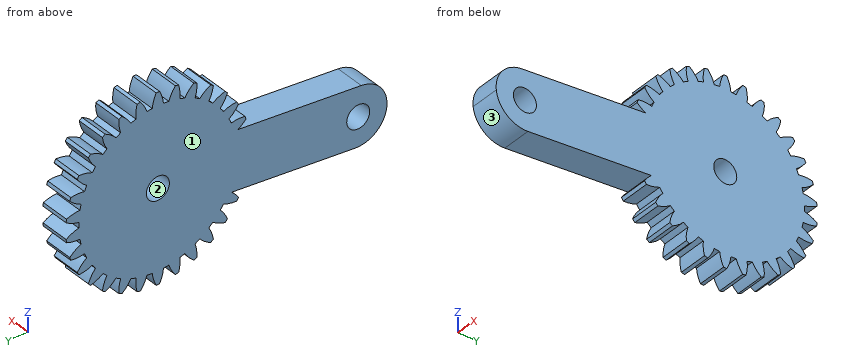
```python
from build123d import *

# Parameters (mm, degrees)
BASPROSKE_W         = 5
BASPROSKE_H         = 16
TOOTHCUT_DEPTH      = 24.173260453
TEETHCUTS_COUNT     = 30
TEETHCUTS_ANGLE     = 348
BORSKE_R            = 0.4
BORE_DEPTH          = 50.0000508
SKETCH1_R           = 2
BOSS_EXTRUDE1_DEPTH = 5
SKETCH2_R           = 2
CUT_EXTRUDE1_DEPTH  = 44.650585033
FILLET1_R           = 5


with BuildPart() as part:
    # BasProSke → Base-Revolve (revolve)
    with BuildSketch(Plane(origin=(0, 0, 0), x_dir=(1, 0, 0), z_dir=(0, 1, 0)), mode=Mode.PRIVATE) as base_revolve_sk:
        with Locations((2.5, 8)):
            Rectangle(BASPROSKE_W, BASPROSKE_H)
    revolve(base_revolve_sk.sketch.rotate(Axis((-10, 0, 0), (1, 0, 0)), 180), axis=Axis((-10, 0, 0), (1, 0, 0)))

    # TooCutSke → ToothCut (cut, through all)
    with BuildSketch(Plane(origin=(0, 0, 0), x_dir=(0, 0, -1), z_dir=(1, 0, 0))):
        with BuildLine():
            ThreePointArc((0.466400716, 13.741086979), (0, 13.749), (-0.466400716, 13.741086979))
            ThreePointArc((-0.466400716, 13.741086979), (-0.819142092, 14.899954875), (-1.3974676, 15.964351834))
            ThreePointArc((-1.3974676, 15.964351834), (0, 16.0254), (1.3974676, 15.964351834))
            ThreePointArc((1.3974676, 15.964351834), (0.819142092, 14.899954875), (0.466400716, 13.741086979))
        make_face()
    toothcut = extrude(amount=TOOTHCUT_DEPTH, mode=Mode.SUBTRACT)

    # TeethCuts: ToothCut ×30 about axis
    teethcuts_axis = Axis((-10, 0, 0), (1, 0, 0))
    for i in range(1, TEETHCUTS_COUNT):
        add(toothcut.rotate(teethcuts_axis, i * TEETHCUTS_ANGLE / (TEETHCUTS_COUNT - 1)), mode=Mode.SUBTRACT)

    # BorSke → Bore (cut, symmetric)
    with BuildSketch(Plane(origin=(0, 0, 0), x_dir=(0, 0, -1), z_dir=(1, 0, 0))):
        with Locations(Location((0, 0, 0), (0, 0, 180))):
            Circle(BORSKE_R)
    extrude(amount=BORE_DEPTH, both=True, mode=Mode.SUBTRACT)

    # Sketch1 → Boss-Extrude1 (add)
    with BuildSketch(Plane(origin=(5, 0, 0), x_dir=(0, 0, -1), z_dir=(1, 0, 0))):
        Polygon((4.972609477, 0.522642316), (9.153748008, -39.258233498), (-0.791470946, -40.303518131), (-4.972609477, -0.522642316), align=None)
        with Locations((3.658496214, -34.808266338)):
            Circle(SKETCH1_R, mode=Mode.SUBTRACT)
    extrude(amount=-BOSS_EXTRUDE1_DEPTH)

    # Sketch2 → Cut-Extrude1 (cut, through all)
    with BuildSketch(Plane(origin=(5, 0, 0), x_dir=(0, 0, -1), z_dir=(1, 0, 0))):
        Circle(SKETCH2_R)
    extrude(amount=-CUT_EXTRUDE1_DEPTH, mode=Mode.SUBTRACT)

    # Fillet1
    fillet1_edges = [part.edges().sort_by_distance(p)[0] for p in [
        (2.5, -39.258233498, -9.153748008),
        (2.5, -40.303518131, 0.791470946),
    ]]
    fillet(fillet1_edges, radius=FILLET1_R - 0.0001)  # a hair under: the kernel refuses the full size


solid = part.part
```
Here's how the part is built. I have some questions about the finished solid (model axes, mm). Face numbers are marked on the shaded views. Coordinates: 2 decimals unless noted, no trailing zeros. Order: outer loops, then holes, each group sorted by start corner. A loop starts at its lowest first (then second) coordinate and runs counter-clockwise, first axis right, second up. Notation, with made-up numbers: (80, 41.5) -> (133, 41.5) arc R16 ccw to (133, 66.5) -> close; hole circle Ø7 at (44, 25). An arc over 180 degrees is marked (long way). Return JSON: item names as keys, results as strings.
1) If we section it at A-A on x = 3.2: State how many separate pieces and enclosed holes the cut face has, plus the area to 3 significant figures.
Conclusion:
{"separate pieces": "1", "enclosed holes": "2", "area": "910 mm²"}
2) I'm going to push flat-ended pins straight in: P1, Ø3, axis at x = 1, y = 2.5, coming from the +Z side; P2, Ø2, axis at x = 2, z = 7, coming from the +Y side; P3, Ø3, axis at y = 0, z = 0, coming from the +X side. Where does each tip first touch, or does it pass through?
Conclusion:
{"P1": "stops at z = 15.71", "P2": "stops at y = 14", "P3": "passes through"}
3) If I drill on probe 1 along Y at (x, z) = (2.9, 14); probe 2 along Z at (x, y) = (0.3, -12); probe 3 along Y at (x, z) = (1.5, 0), over which ranges is the centre line in solid material (lowest first)?
Conclusion:
{"probe 1": "y = -6.79 to -5.46, -3.85 to -2.03, -0.94 to 0.94, 2.03 to 3.85, 5.46 to 6.79", "probe 2": "z = -10.58 to -10.27, -7.94 to 7.94, 10.27 to 10.58", "probe 3": "y = -38.22 to -2, 2 to 13.75"}
4) Thinking about a two-plate mould opening in Z: for the marked faces 1, 2 and 3, which applies, +Z half, -Z half, draft (parallel to the pull), parting line (faces both ways), or undercut?
Conclusion:
{"face 1": "draft", "face 2": "undercut", "face 3": "-Z half"}
5) If we section it at B-B on y = -26.5: List the corners of the cut face in (x, z) for me, plus the area to 3 significant figures.
Conclusion:
{"outline": "(0, -7.81) -> (5, -7.81) -> (5, 2.24) -> (0, 2.24) -> close", "area": "50.3 mm²"}
